Read the model definition and answer for the solid it produces. Units are mm, in the model's axes. Face numbers are marked on the shaded views. A direction names the side the tool comes from. Coordinates: 2 decimals unless noted, no trailing zeros. Loops run counter-clockwise (first coordinate to the right, second up) from the corner with the lowest first, then second, coordinate; pieces in that order, holes last. Notation, with made-up numbers: M 6.5,51 L 11.5,51 A28 ccw 11.5,74 Z; hole C 61.5,66.5 d8. An arc over 180 degrees is marked long. Put each result on its own line as item: value.
from build123d import *

# Parameters (mm, degrees)
SKETCH1_R           = 1.9
BOSS_EXTRUDE1_DEPTH = 2
BOSS_EXTRUDE2_START = 1
SKETCH2_R           = 1
BOSS_EXTRUDE2_DEPTH = 1
SKETCH3_W           = 7.26
SKETCH3_H           = 2.991248821
CUT_EXTRUDE1_DEPTH  = 10
FILLET1_R           = 1


with BuildPart() as part:
    # Sketch1 → Boss-Extrude1 (new body)
    with BuildSketch(Plane.XY):
        with BuildLine():
            Line((1, 0), (19.26, 0))
            ThreePointArc((19.26, 0), (19.967106781, 0.292893219), (20.26, 1))
            Line((20.26, 1), (20.26, 4.371699928))
            ThreePointArc((20.26, 4.371699928), (19.967106781, 5.078806709), (19.26, 5.371699928))
            Line((19.26, 5.371699928), (1, 5.371699928))
            ThreePointArc((1, 5.371699928), (0.292893219, 5.078806709), (0, 4.371699928))
            Line((0, 4.371699928), (0, 1))
            ThreePointArc((0, 1), (0.292893219, 0.292893219), (1, 0))
        make_face()
        with Locations((3, 2.685849964)):
            Circle(SKETCH1_R, mode=Mode.SUBTRACT)
        with Locations((17.26, 2.685849964)):
            Circle(SKETCH1_R, mode=Mode.SUBTRACT)
    extrude(amount=BOSS_EXTRUDE1_DEPTH)

    # Sketch2 → Boss-Extrude2 (add)
    with BuildSketch(Plane(origin=(0, 0, 0), x_dir=(-1, 0, 0), z_dir=(0, 0, -1)).offset(BOSS_EXTRUDE2_START)):
        with BuildLine():
            Line((-19.26, 0), (-1, 0))
            ThreePointArc((-1, 0), (-0.292893219, 0.292893219), (0, 1))
            Line((0, 1), (0, 4.371699928))
            ThreePointArc((0, 4.371699928), (-0.292893219, 5.078806709), (-1, 5.371699928))
            Line((-1, 5.371699928), (-19.26, 5.371699928))
            ThreePointArc((-19.26, 5.371699928), (-19.967106781, 5.078806709), (-20.26, 4.371699928))
            Line((-20.26, 4.371699928), (-20.26, 1))
            ThreePointArc((-20.26, 1), (-19.967106781, 0.292893219), (-19.26, 0))
        make_face()
        with Locations((-17.26, 2.685849964)):
            Circle(SKETCH2_R, mode=Mode.SUBTRACT)
        with Locations((-3, 2.685849964)):
            Circle(SKETCH2_R, mode=Mode.SUBTRACT)
    extrude(amount=-BOSS_EXTRUDE2_DEPTH)

    # Sketch3 → Cut-Extrude1 (cut)
    with BuildSketch(Plane.XZ):
        with Locations((10.13, 2.495624411)):
            Rectangle(SKETCH3_W, SKETCH3_H)
    extrude(amount=-CUT_EXTRUDE1_DEPTH, mode=Mode.SUBTRACT)

    # Fillet1
    fillet1_edges = [part.edges().sort_by_distance(p)[0] for p in [
        (13.76, 2.685849964, 2),
        (6.5, 2.685849964, 2),
    ]]
    fillet(fillet1_edges, radius=FILLET1_R - 0.0001)  # a hair under: the kernel refuses the full size


solid = part.part
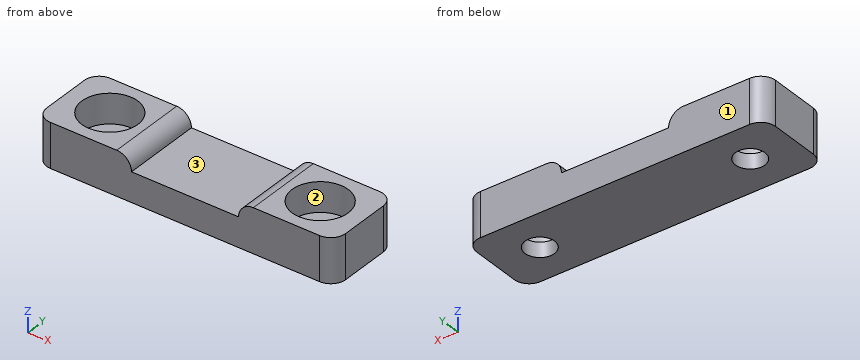
1) Find section A-A, the plane x = 3. Write down the section's boundary in (y, z).
Answer list:
outline: M 0,-1 L 1.69,-1 L 1.69,0 L 0.79,0 L 0.79,2 L 0,2 Z; M 3.69,-1 L 5.37,-1 L 5.37,2 L 4.59,2 L 4.59,0 L 3.69,0 Z
2) Find section B-B, the plane z = 1.25. Write down the section's boundary in (x, y), plus the area to 3 significant figures.
Answer list:
outline: M 0,1 A1 ccw 1,0 L 6.47,0 L 6.47,5.37 L 1,5.37 A1 ccw 0,4.37 Z; M 13.79,0 L 19.26,0 A1 ccw 20.26,1 L 20.26,4.37 A1 ccw 19.26,5.37 L 13.79,5.37 Z; hole C 3,2.69 d3.8; hole C 17.26,2.69 d3.8
area: 46.0 mm^2
3) Straight lines are drawn through the part: line 1 (Y direction, x = 3, z = 0.6); line 2 (X direction, y = 1.45, z = 0.1); line 3 (X direction, y = 1.2, z = 1.5). For each, find the intervals that lie inside material, in ascending order. Write a range as [from, to].
Answer list:
line 1: y = [0, 0.79], [4.59, 5.37]
line 2: x = [0, 1.56], [4.44, 15.82], [18.7, 20.26]
line 3: x = [0, 1.82], [4.18, 6.37], [13.89, 16.08], [18.44, 20.26]
4) Find section D-D, the plane z = -0.5. Write down the section's boundary in (x, y), plus the area to 3 significant figures.
Answer list:
outline: M 0,1 A1 ccw 1,0 L 19.26,0 A1 ccw 20.26,1 L 20.26,4.37 A1 ccw 19.26,5.37 L 1,5.37 A1 ccw 0,4.37 Z; hole C 3,2.69 d2; hole C 17.26,2.69 d2
area: 102 mm^2
5) Given pin 1 Ø1 at (y, z) = (0.5, 1) entering from +X; pin 2 Ø1.8 at (x, y) = (17.26, 2.69) entering from -Z, each flat-ended and moving along its own axis, determine where each tip first touches the part or whether it passes through.
Answer list:
pin 1: stops at x = 20.26
pin 2: passes through
6) Which of the six approach directions +Z, -Z, +X, -X, +Y, -Y give full straight-line access (tool end or side, diameter ignored) to the marked faces 1, 2 and 3?
Answer list:
face 1: +Z, -Z, +X, -X, +Y
face 2: +Z
face 3: +Z, +Y, -Y
7) Find section C-C, the plane y = 1.9. Count the separate pieces of the cut face and the enclosed holes in it, plus the area to 3 significant figures.
Answer list:
separate pieces: 3
enclosed holes: 0
area: 36.8 mm^2
